from build123d import *

# Parameters (mm, degrees)
SKETCH1_W               = 130
SKETCH1_H               = 120
BOSS_EXTRUDE1_DEPTH     = 3
CUT_EXTRUDE1_START      = -4
SKETCH2_W               = 20
SKETCH2_H               = 89
CUT_EXTRUDE1_DEPTH      = 5
CUT_EXTRUDE2_START      = -4
SKETCH3_R               = 1.6
CUT_EXTRUDE2_DEPTH      = 5
SKETCH4_W               = 130
SKETCH4_H               = 82
CUT_EXTRUDE3_DEPTH      = 1
CUT_EXTRUDE3_DEPTH_BACK = 4


with BuildPart() as part:
    # Sketch1 → Boss-Extrude1 (new body)
    with BuildSketch(Plane(origin=(0, 0, 0), x_dir=(1, 0, 0), z_dir=(0, 1, 0))):
        Rectangle(SKETCH1_W, SKETCH1_H)
    extrude(amount=BOSS_EXTRUDE1_DEPTH)

    # Sketch2 → Cut-Extrude1 (cut)
    with BuildSketch(Plane(origin=(0, 3, 0), x_dir=(1, 0, 0), z_dir=(0, 1, 0)).offset(CUT_EXTRUDE1_START)):
        with Locations((-16.25, 0)):
            Rectangle(SKETCH2_W, SKETCH2_H)
    cut_extrude1 = extrude(amount=CUT_EXTRUDE1_DEPTH, mode=Mode.SUBTRACT)

    # Mirror1: Cut-Extrude1 across plane
    add(cut_extrude1.mirror(Plane(origin=(0, 0, 0), x_dir=(0, 0, 1), z_dir=(1, 0, 0))), mode=Mode.SUBTRACT)

    # Sketch3 → Cut-Extrude2 (cut)
    with BuildSketch(Plane(origin=(0, 3, 0), x_dir=(1, 0, 0), z_dir=(0, 1, 0)).offset(CUT_EXTRUDE2_START)):
        with Locations((44.5, 0)):
            Circle(SKETCH3_R)
    cut_extrude2 = extrude(amount=CUT_EXTRUDE2_DEPTH, mode=Mode.SUBTRACT)

    # Mirror2: Cut-Extrude2 across plane
    add(cut_extrude2.mirror(Plane(origin=(0, 0, 0), x_dir=(0, 0, 1), z_dir=(1, 0, 0))), mode=Mode.SUBTRACT)

    # Sketch4 → Cut-Extrude3 (cut, two sides)
    with BuildSketch(Plane(origin=(0, 3, 0), x_dir=(1, 0, 0), z_dir=(0, 1, 0))) as cut_extrude3_sk:
        with Locations((0, 19)):
            Rectangle(SKETCH4_W, SKETCH4_H)
    extrude(amount=CUT_EXTRUDE3_DEPTH, mode=Mode.SUBTRACT)
    extrude(cut_extrude3_sk.sketch, amount=-CUT_EXTRUDE3_DEPTH_BACK, mode=Mode.SUBTRACT)


solid = part.part
Verification items for the finished model (mm, model axes). A direction names the side the tool comes from. Give positions to 0.01 mm unless a question says otherwise; leave off trailing zeros. Write each loop counter-clockwise with the first axis right and the second up, starting at its lowest first coordinate (ties: lowest second). Pieces come first, ordered by that corner, then holes.
(1) Cross-section at C-C (x = 14). Enter the section's corners in (y, z), plus the area to 3 significant figures.
(2) Material ranges on line 1 (X direction, y = 1.15, z = 33.5); line 2 (Z direction, x = -19.5, y = 1.4), recorded low to high.
(3) Cross-section at B-B (y = 2.55). Enter the section's corners in (x, z).
(4) Access from +Z, -Z, +X, -X, +Y, -Y to the whole of each face (thin tool, end or side, straight path). Record for faces 1 (the face through (26.25, 1, 33)), 2 (the face through (45, 2, 22)).
(5) Cross-section at A-A (z = 36). Enter the section's corners in (x, y).
(6) Mould release check, pull along X, two halves, no side actions. Record for faces 3 (the face through (-26.25, 1, 33)), 4 (the face through (-65, 1, 41)), 5 (the face through (65, 1, 41)): +X half, -X half, draft (parallel to the pull), parting line (faces both ways), or undercut.
Worked out:
1. outline: (0, 44.5) - (3, 44.5) - (3, 60) - (0, 60) - close
1. area: 46.5 mm2
2. line 1: x = -65 to -26.25, -6.25 to 6.25, 26.25 to 65
2. line 2: z = 44.5 to 60
3. outline: (-65, 22) - (-26.25, 22) - (-26.25, 44.5) - (-6.25, 44.5) - (-6.25, 22) - (6.25, 22) - (6.25, 44.5) - (26.25, 44.5) - (26.25, 22) - (65, 22) - (65, 60) - (-65, 60) - close
4. face 1: -Z, +Y, -Y
4. face 2: -Z, +X, -X, +Y, -Y
5. outline: (-65, 0) - (-26.25, 0) - (-26.25, 3) - (-65, 3) - close; (-6.25, 0) - (6.25, 0) - (6.25, 3) - (-6.25, 3) - close; (26.25, 0) - (65, 0) - (65, 3) - (26.25, 3) - close
6. face 3: undercut
6. face 4: -X half
6. face 5: +X half
